Work out the finished part from the listing and answer in its coordinate system (mm). A direction names the side the tool comes from. Give positions to 0.01 mm unless a question says otherwise; leave off trailing zeros. Loops run counter-clockwise (first coordinate to the right, second up) from the corner with the lowest first, then second, coordinate; pieces in that order, holes last. Notation, with made-up numbers: M 45.25,79.25 L 54.25,79.25 A16 ccw 54.25,93.25 Z; hole C -11.5,32 d7. An arc over 180 degrees is marked long. Answer in a Markdown table with one row per item. Add a question column.
from build123d import *

# Parameters (mm, degrees)
SKETCH1_W           = 35
SKETCH1_H           = 10
BOSS_EXTRUDE1_DEPTH = 1.5
SKETCH2_R           = 1.65
CUT_EXTRUDE1_DEPTH  = 3
SKETCH3_W           = 18
SKETCH3_H           = 10
BOSS_EXTRUDE2_DEPTH = 54


with BuildPart() as part:
    # Sketch1 → Boss-Extrude1 (new body, symmetric)
    with BuildSketch(Plane(origin=(0, 0, 0), x_dir=(1, 0, 0), z_dir=(0, 1, 0))):
        Rectangle(SKETCH1_W, SKETCH1_H)
    boss_extrude1 = extrude(amount=BOSS_EXTRUDE1_DEPTH, both=True)

    # Sketch2 → Cut-Extrude1 (cut)
    with BuildSketch(Plane(origin=(0, 1.5, 0), x_dir=(1, 0, 0), z_dir=(0, 1, 0))):
        with Locations((-13.5, 1)):
            Circle(SKETCH2_R)
        with Locations((13.5, 1)):
            Circle(SKETCH2_R)
    cut_extrude1 = extrude(amount=-CUT_EXTRUDE1_DEPTH, mode=Mode.SUBTRACT)

    # Sketch3 → Boss-Extrude2 (add)
    with BuildSketch(Plane(origin=(0, 1.5, 0), x_dir=(1, 0, 0), z_dir=(0, 1, 0))):
        Rectangle(SKETCH3_W, SKETCH3_H)
    extrude(amount=BOSS_EXTRUDE2_DEPTH)

    # Mirror1: Boss-Extrude1, Cut-Extrude1 across plane
    add(boss_extrude1.mirror(Plane.ZX.offset(28.5)))
    add(cut_extrude1.mirror(Plane.ZX.offset(28.5)), mode=Mode.SUBTRACT)


solid = part.part
(1) Section C-C, the plane x = 13.5 is taken. Determine the outline of the cut face in (y, z), and give its area (3 significant figures).
(2) The mould has two halves that part along X. Classify faces 4 (the face through (17.5, 0, 0)), 5 (the face through (15.024, 56.979, -0.368)), 6 (the face through (-9, 28, 0)): pulls with the +X half, pulls with the -X half, needs draft (parallel to the pull), parting line crosses it, or undercut.
(3) Which of the six approach directions +Z, -Z, +X, -X, +Y, -Y give full straight-line access (tool end or side, diameter ignored) to faces 1 (the face through (13, 55.5, 1)), 2 (the face through (0, 28, -5)), 3 (the face through (-13, 55.5, 1))?
(4) Section D-D, the plane z = 4 is taken. Determine the outline of the cut face in (x, y).
(5) Section B-B, the plane z = -1 is taken. Determine the outline of the cut face in (x, y).
(6) Consider line 1 along X through (y, z) = (57.45, -1); line 2 along Z through (x, y) = (-13.5, 0.4); line 3 along Y through (x, z) = (12.5, -3.5). Determine where each line is inside the solid, lowest interval first. Write a range as from..to.
(7) Section A-A, the plane x = 10 is taken. Determine the outline of the cut face in (y, z).
(8) This flat-tipped pin is pushed along its axis until it touches: P1, Ø5, axis at y = 7, z = 3.5, coming from the -X side. Where does it stop, or does it pass through?
Numbers:
| question | item | result |
|---|---|---|
| 1 | outline | M -1.5,-5 L 1.5,-5 L 1.5,-2.65 L -1.5,-2.65 Z; M -1.5,0.65 L 1.5,0.65 L 1.5,5 L -1.5,5 Z; M 55.5,-5 L 58.5,-5 L 58.5,-2.65 L 55.5,-2.65 Z; M 55.5,0.65 L 58.5,0.65 L 58.5,5 L 55.5,5 Z |
| 1 | area | 40.2 mm² |
| 2 | face 4 | pulls with the +X half |
| 2 | face 5 | undercut |
| 2 | face 6 | pulls with the -X half |
| 3 | face 1 | +Z, -Z, +X |
| 3 | face 2 | -Z, +X, -X, +Y, -Y |
| 3 | face 3 | +Z, -Z, -X |
| 4 | outline | M -17.5,-1.5 L 17.5,-1.5 L 17.5,1.5 L 9,1.5 L 9,55.5 L 17.5,55.5 L 17.5,58.5 L -17.5,58.5 L -17.5,55.5 L -9,55.5 L -9,1.5 L -17.5,1.5 Z |
| 5 | outline | M -17.5,-1.5 L -15.15,-1.5 L -15.15,1.5 L -17.5,1.5 Z; M -17.5,55.5 L -15.15,55.5 L -15.15,58.5 L -17.5,58.5 Z; M -11.85,-1.5 L 11.85,-1.5 L 11.85,1.5 L 9,1.5 L 9,55.5 L 11.85,55.5 L 11.85,58.5 L -11.85,58.5 L -11.85,55.5 L -9,55.5 L -9,1.5 L -11.85,1.5 Z; M 15.15,-1.5 L 17.5,-1.5 L 17.5,1.5 L 15.15,1.5 Z; M 15.15,55.5 L 17.5,55.5 L 17.5,58.5 L 15.15,58.5 Z |
| 6 | line 1 | x = -17.5..-15.15, -11.85..11.85, 15.15..17.5 |
| 6 | line 2 | z = -5..-2.65, 0.65..5 |
| 6 | line 3 | y = -1.5..1.5, 55.5..58.5 |
| 7 | outline | M -1.5,-5 L 1.5,-5 L 1.5,5 L -1.5,5 Z; M 55.5,-5 L 58.5,-5 L 58.5,5 L 55.5,5 Z |
| 8 | P1 | stops at x = -9 |
